from build123d import *

# Parameters (mm, degrees)
BOSS_EXTRUDE1_DEPTH = 3
CUT_EXTRUDE1_DEPTH  = 128.25921375
LPATTERN1_COUNT     = 4
LPATTERN1_PITCH     = 35
CUT_EXTRUDE3_DEPTH  = 3
LPATTERN2_COUNT     = 3
LPATTERN2_PITCH     = 35
CUT_EXTRUDE4_DEPTH  = 3
LPATTERN3_COUNT     = 3
LPATTERN3_PITCH     = 35
CAVITY1_START       = -7.796688406
CAVITY1_DEPTH       = 3


# Read off the part's stored shape, not the designer's step: Cavity1
with BuildPart() as part:
    # Sketch1 → Boss-Extrude1 (new body)
    with BuildSketch(Plane.XY):
        Polygon((-63.438534121, 102.766276007), (63.438534121, 102.766276007), (75, -7.839634745), (-75, -7.839634745), align=None)
    extrude(amount=BOSS_EXTRUDE1_DEPTH)

    # Sketch2 → Cut-Extrude1 (cut, symmetric)
    with BuildSketch(Plane.XY):
        Polygon((-56.956577019, 457.127747207), (-56.956577019, 102.766276007), (-56.956577019, 99.766276007), (-46.956577019, 99.766276007), (-46.956577019, 102.766276007), (-46.956577019, 457.127747207), (-46.956577019, 1165.850689606), (-56.956577019, 1165.850689606), align=None)
    cut_extrude1 = extrude(amount=CUT_EXTRUDE1_DEPTH, both=True, mode=Mode.SUBTRACT)

    # LPattern1: Cut-Extrude1 ×4
    with Locations(*[(i * LPATTERN1_PITCH, 0, 0) for i in range(1, LPATTERN1_COUNT)]):
        add(cut_extrude1, mode=Mode.SUBTRACT)

    # Sketch3 → Cut-Extrude3 (cut)
    with BuildSketch(Plane.XY.offset(3)):
        Polygon((-74.180535028, 0), (-71.180535028, 0), (-70.140914516, 9.945812646), (-73.140914516, 9.945812646), align=None)
    cut_extrude3 = extrude(amount=-CUT_EXTRUDE3_DEPTH, mode=Mode.SUBTRACT)

    # LPattern2: Cut-Extrude3 ×3
    with Locations(*[Vector(0.10396205118449778, 0.9945812646101434, 0) * (i * LPATTERN2_PITCH) for i in range(1, LPATTERN2_COUNT)]):
        add(cut_extrude3, mode=Mode.SUBTRACT)

    # Sketch7 → Cut-Extrude4 (cut)
    with BuildSketch(Plane.XY.offset(3)):
        Polygon((74.180535028, 0), (73.140914516, 9.945812646), (70.157170722, 9.633926493), (71.196791234, -0.311886154), align=None)
    cut_extrude4 = extrude(amount=-CUT_EXTRUDE4_DEPTH, mode=Mode.SUBTRACT)

    # LPattern3: Cut-Extrude4 ×3
    with Locations(*[Vector(-0.10396205118449776, 0.9945812646101434, 0) * (i * LPATTERN3_PITCH) for i in range(1, LPATTERN3_COUNT)]):
        add(cut_extrude4, mode=Mode.SUBTRACT)

    # Cavity1 outline → Cavity1 (cut)
    with BuildSketch(Plane(origin=(0, 0, 0), x_dir=(1, 0, 0), z_dir=(0, 0.9945218953682734, -0.10452846326765304)).offset(CAVITY1_START)):
        Polygon((-56.749963879, 2), (-56.749963879, -2.180535028), (-66.749963879, -2.180535028), (-66.749963879, 2), (-77, 2), (-77, -4), (77, -4), (77, 2), (63.250036121, 2), (63.250036121, -2.180535028), (53.250036121, -2.180535028), (53.250036121, 2), (33.250036121, 2), (33.250036121, -2.180535028), (23.250036121, -2.180535028), (23.250036121, 2), (3.250036121, 2), (3.250036121, -2.180535028), (-6.749963879, -2.180535028), (-6.749963879, 2), (-26.749963879, 2), (-26.749963879, -2.180535028), (-36.749963879, -2.180535028), (-36.749963879, 2), align=None)
    extrude(amount=CAVITY1_DEPTH, mode=Mode.SUBTRACT)


solid = part.part
Build history of the part. All positions in model axes, mm. A direction names the side the tool comes from. Round coordinates to 2 decimals unless told otherwise and drop trailing zeros. Loops run counter-clockwise (first coordinate to the right, second up) from the corner with the lowest first, then second, coordinate; pieces in that order, holes last. Notation, with made-up numbers: (41, -39.75) -> (82, -39.75) arc R11 cw to (82, -32.75) -> close; hole circle Ø1 at (-21.5, -13.5). An arc over 180 degrees is marked (long way). Use CSV: the item, a comma, the result in double quotes. Start each with the question number.
Q1. Saw through at B-B on z = 1.7. Count the separate pieces of the cut face and the enclosed holes in it, and give its area (3 significant figures).
Q2. Mould opens along Y. For faces 4 (the face through (1, -7.84, 1)), 5 (the face through (18, 99.766, 2)), 6 (the face through (63.25, -6, 1)) say: +Y half, -Y half, draft (parallel to the pull), parting line (faces both ways), or undercut.
Q3. Saw through at C-C on y = 90. Give the cut face in (x, z).
Q4. Drill centre lines: L1, parallel to Y at x = 54, z = 2.15; L2, parallel to Y at x = -19.5, z = 2.7; L3, parallel to Y at x = -53.5, z = 2. Where is each one in solid material? Low to high.
Q5. Saw through at D-D on y = 11.5. Give the cut face in (x, z), and give its area (3 significant figures).
Q6. Which spindle directions (+Z, -Z, +X, -X, +Y, -Y) get a long thin tool onto all of the face, cutting with end or side? Do faces 1 (the face through (-11.957, 101, 2)), 2 (the face through (-65, 69.621, 2)), 3 (the face through (69.029, 34.652, 1.521)). Say none if no direction does.
Q7. Saw through at A-A on x = 45. Give the cut face in (y, z), and give its area (3 significant figures).
Q8. Flat gauge pins, fed straight in: pin 1 Ø0.9 at (y, z) = (-5.5, 2) entering from -X; pin 2 Ø1.5 at (y, z) = (101.5, 1) entering from -X; pin 3 Ø1.5 at (x, z) = (14, 1.5) entering from +Y. Where does each tip first touch, or does it go through?
Solutions:
1,separate pieces,"1"
1,enclosed holes,"4"
1,area,"14,700 mm^2"
2,face 4,"-Y half"
2,face 5,"+Y half"
2,face 6,"undercut"
3,outline,"(-64.77, 0) -> (64.77, 0) -> (64.77, 3) -> (-64.77, 3) -> close"
4,L1,"y = -7.84 to 99.77"
4,L2,"y = -7.84 to -7.56, -4.54 to 99.77"
4,L3,"y = -7.84 to -7.63, -4.61 to 99.77"
5,outline,"(-72.98, 0) -> (72.98, 0) -> (72.98, 3) -> (-72.98, 3) -> close"
5,area,"438 mm^2"
6,face 1,"+Z, -Z, +Y"
6,face 2,"+Z, -Z, -X"
6,face 3,"+Z, -Z"
7,outline,"(-7.84, 0) -> (-7.52, 3) -> (-7.84, 3) -> close; (-4.82, 0) -> (102.77, 0) -> (102.77, 3) -> (-4.51, 3) -> close"
7,area,"323 mm^2"
8,pin 1,"stops at x = -66.75"
8,pin 2,"stops at x = -63.65"
8,pin 3,"stops at y = 99.77"
